```python
from build123d import *

# Parameters (mm, degrees)
BOSS_EXTRUDE1_DEPTH              = 3.7
CUT_EXTRUDE1_DEPTH               = 1.2
CUT_EXTRUDE2_DEPTH               = 2
CUT_EXTRUDE3_DEPTH               = 20.027535968
BOSS_EXTRUDE3_DEPTH              = 5
M2_CLEARANCE_HOLE1_D             = 2.6
CUT_EXTRUDE4_DEPTH               = 1
CHAMFER2_SIZE                    = 0.75
BOSS_EXTRUDE4_DEPTH              = 3
BOSS_EXTRUDE5_START              = 3
BOSS_EXTRUDE5_DEPTH              = 3
CBORE_FOR_M2_5_SHCS1_D           = 3.1
CBORE_FOR_M2_5_SHCS1_CBORE_D     = 5.5
CBORE_FOR_M2_5_SHCS1_CBORE_DEPTH = 1.5
CUT_EXTRUDE6_DEPTH               = 2.5
SKETCH18_R                       = 3.62
CUT_EXTRUDE7_DEPTH               = 1
CBORE_FOR_M2_SHCS1_D             = 2.6
CBORE_FOR_M2_SHCS1_CBORE_D       = 4.4
CBORE_FOR_M2_SHCS1_CBORE_DEPTH   = 1.5
CHAMFER3_SIZE                    = 0.5
BOSS_EXTRUDE8_DEPTH              = 7.5
BOSS_EXTRUDE9_DEPTH              = 6
FILLET1_R                        = 1


with BuildPart() as part:
    # Sketch1 → Boss-Extrude1 (new body)
    with BuildSketch(Plane(origin=(0, -6, 0), x_dir=(-1, 0, 0), z_dir=(0, -1, 0))):
        with BuildLine():
            Line((7.595, 10.65), (-7.595, 10.65))
            ThreePointArc((-7.595, 10.65), (-11.604295449, 8.989295449), (-13.265, 4.98))
            Line((-13.265, 4.98), (-13.265, -7.46))
            ThreePointArc((-13.265, -7.46), (-11.604295449, -11.469295449), (-7.595, -13.13))
            Line((-7.595, -13.13), (7.595, -13.13))
            ThreePointArc((7.595, -13.13), (11.604295449, -11.469295449), (13.265, -7.46))
            Line((13.265, -7.46), (13.265, 4.98))
            ThreePointArc((13.265, 4.98), (11.604295449, 8.989295449), (7.595, 10.65))
        make_face()
    extrude(amount=-BOSS_EXTRUDE1_DEPTH)

    # Sketch3 → Cut-Extrude1 (cut)
    with BuildSketch(Plane(origin=(0, -2.3, 0), x_dir=(1, 0, 0), z_dir=(0, 1, 0))):
        with BuildLine():
            Line((-7.595, -10.48), (7.595, -10.48))
            ThreePointArc((7.595, -10.48), (9.730462479, -9.595462479), (10.615, -7.46))
            Line((10.615, -7.46), (10.615, 4.98))
            ThreePointArc((10.615, 4.98), (9.730462479, 7.115462479), (7.595, 8))
            Line((7.595, 8), (-7.595, 8))
            ThreePointArc((-7.595, 8), (-9.730462479, 7.115462479), (-10.615, 4.98))
            Line((-10.615, 4.98), (-10.615, -7.46))
            ThreePointArc((-10.615, -7.46), (-9.730462479, -9.595462479), (-7.595, -10.48))
        make_face()
    extrude(amount=-CUT_EXTRUDE1_DEPTH, mode=Mode.SUBTRACT)

    # Sketch4 → Cut-Extrude2 (cut)
    with BuildSketch(Plane(origin=(0, -6, 0), x_dir=(1, 0, 0), z_dir=(0, 1, 0))):
        with BuildLine():
            Line((9.25, -4.27), (-9.25, -4.27))
            ThreePointArc((-9.25, -4.27), (-9.603553391, -4.416446609), (-9.75, -4.77))
            Line((-9.75, -4.77), (-9.75, -11.98))
            Line((-9.75, -11.98), (-9.75, -13.13))
            Line((-9.75, -13.13), (9.75, -13.13))
            Line((9.75, -13.13), (9.75, -11.98))
            Line((9.75, -11.98), (9.75, -4.77))
            ThreePointArc((9.75, -4.77), (9.603553391, -4.416446609), (9.25, -4.27))
        make_face()
    extrude(amount=CUT_EXTRUDE2_DEPTH, mode=Mode.SUBTRACT)

    # Sketch5 → Cut-Extrude3 (cut, through all)
    with BuildSketch(Plane(origin=(0, -2.3, 0), x_dir=(1, 0, 0), z_dir=(0, 1, 0))):
        with BuildLine():
            Line((-9.25, -9.63), (9.25, -9.63))
            ThreePointArc((9.25, -9.63), (9.603553391, -9.483553391), (9.75, -9.13))
            Line((9.75, -9.13), (9.75, -4.77))
            ThreePointArc((9.75, -4.77), (9.603553391, -4.416446609), (9.25, -4.27))
            Line((9.25, -4.27), (-9.25, -4.27))
            ThreePointArc((-9.25, -4.27), (-9.603553391, -4.416446609), (-9.75, -4.77))
            Line((-9.75, -4.77), (-9.75, -9.13))
            ThreePointArc((-9.75, -9.13), (-9.603553391, -9.483553391), (-9.25, -9.63))
        make_face()
    extrude(amount=-CUT_EXTRUDE3_DEPTH, mode=Mode.SUBTRACT)

    # Sketch6 → Boss-Extrude3 (add, symmetric)
    with BuildSketch(Plane(origin=(0, 0, 1.24), x_dir=(-1, 0, 0), z_dir=(0, 0, -1))):
        Polygon((-11.94, -2.3), (-11.94, 0.7), (-11.44, 0.7), (-11.44, 1.7), (-12.19, 2.45), (-13.265, 2.45), (-13.265, -2.3), align=None)
    boss_extrude3 = extrude(amount=BOSS_EXTRUDE3_DEPTH, both=True)

    # Mirror1: Boss-Extrude3 across plane
    add(boss_extrude3.mirror(Plane(origin=(0, 0, 0), x_dir=(0, 0, 1), z_dir=(1, 0, 0))))

    # M2 Clearance Hole1 (through all)
    with Locations(Plane(origin=(0, -3.5, 0), x_dir=(1, 0, 0), z_dir=(0, 1, 0))):
        with Locations((-7.615, 5.15), (7.615, 5.15)):
            Hole(M2_CLEARANCE_HOLE1_D / 2)

    # Sketch9 → Cut-Extrude4 (cut)
    with BuildSketch(Plane.XZ.offset(6)):
        Polygon((-7.615, -2.667393842), (-9.765, -3.908696921), (-9.765, -6.391303079), (-7.615, -7.632606158), (-5.465, -6.391303079), (-5.465, -3.908696921), align=None)
        Polygon((7.615, -2.667393842), (5.465, -3.908696921), (5.465, -6.391303079), (7.615, -7.632606158), (9.765, -6.391303079), (9.765, -3.908696921), align=None)
    extrude(amount=-CUT_EXTRUDE4_DEPTH, mode=Mode.SUBTRACT)

    # Chamfer2
    chamfer2_edges = [part.edges().sort_by_distance(p)[0] for p in [
        (-13.265, 2.45, 1.24),
        (13.265, 2.45, 1.24),
    ]]
    chamfer(chamfer2_edges, length=CHAMFER2_SIZE)

    # Sketch11 → Boss-Extrude4 (add)
    with BuildSketch(Plane(origin=(0, 0, -1.76), x_dir=(-1, 0, 0), z_dir=(0, 0, -1))):
        with BuildLine():
            Line((-16.362587065, -18.187498165), (-0.407985075, -19.601950475))
            ThreePointArc((-0.407985075, -19.601950475), (2.579168763, -18.833052112), (4.416654929, -16.355566021))
            Line((4.416654929, -16.355566021), (7.595, -6))
            Line((7.595, -6), (7.595, -3.5))
            Line((7.595, -3.5), (-7.595, -3.5))
            Line((-7.595, -3.5), (-7.595, -11.035213013))
            Line((-7.595, -11.035213013), (-16.362587065, -11.812501835))
            ThreePointArc((-16.362587065, -11.812501835), (-19.28, -15), (-16.362587065, -18.187498165))
        make_face()
    extrude(amount=-BOSS_EXTRUDE4_DEPTH)

    # Sketch12 → Boss-Extrude5 (add)
    with BuildSketch(Plane(origin=(0, 0, -1.76), x_dir=(-1, 0, 0), z_dir=(0, 0, -1)).offset(BOSS_EXTRUDE5_START)):
        with BuildLine():
            Line((-0.407985075, -10.398049525), (-16.362587065, -11.812501835))
            ThreePointArc((-16.362587065, -11.812501835), (-19.28, -15), (-16.362587065, -18.187498165))
            Line((-16.362587065, -18.187498165), (-0.407985075, -19.601950475))
            ThreePointArc((-0.407985075, -19.601950475), (4.62, -15), (-0.407985075, -10.398049525))
        make_face()
    extrude(amount=-BOSS_EXTRUDE5_DEPTH)

    # CBORE for M2.5 SHCS1 (through all)
    with Locations(Plane.XY.offset(1.24)):
        with Locations((0, -15)):
            CounterBoreHole(CBORE_FOR_M2_5_SHCS1_D / 2, CBORE_FOR_M2_5_SHCS1_CBORE_D / 2, CBORE_FOR_M2_5_SHCS1_CBORE_DEPTH)

    # Sketch17 → Cut-Extrude6 (cut)
    with BuildSketch(Plane(origin=(0, 0, -4.76), x_dir=(-1, 0, 0), z_dir=(0, 0, -1))):
        with BuildLine():
            Line((-0.319676617, -11.394142701), (-16.274278607, -12.808595012))
            ThreePointArc((-16.274278607, -12.808595012), (-18.28, -15), (-16.274278607, -17.191404988))
            Line((-16.274278607, -17.191404988), (-0.319676617, -18.605857299))
            ThreePointArc((-0.319676617, -18.605857299), (3.62, -15), (-0.319676617, -11.394142701))
        make_face()
    extrude(amount=-CUT_EXTRUDE6_DEPTH, mode=Mode.SUBTRACT)

    # Sketch18 → Cut-Extrude7 (cut)
    with BuildSketch(Plane(origin=(0, 0, -2.26), x_dir=(-1, 0, 0), z_dir=(0, 0, -1))):
        with Locations((0, -15)):
            Circle(SKETCH18_R)
    extrude(amount=-CUT_EXTRUDE7_DEPTH, mode=Mode.SUBTRACT)

    # CBORE for M2 SHCS1 (through all)
    with Locations(Plane.XY.offset(1.24)):
        with Locations((14.625, -15)):
            CounterBoreHole(CBORE_FOR_M2_SHCS1_D / 2, CBORE_FOR_M2_SHCS1_CBORE_D / 2, CBORE_FOR_M2_SHCS1_CBORE_DEPTH)

    # Chamfer3
    chamfer3_edges = [part.edges().sort_by_distance(p)[0] for p in [
        (6.54, -6, -3.288045382),
        (8.69, -6, -3.288045382),
        (5.465, -6, -5.15),
        (9.765, -6, -5.15),
        (6.54, -6, -7.011954618),
        (8.69, -6, -7.011954618),
        (-8.69, -6, -3.288045382),
        (-6.54, -6, -3.288045382),
        (-9.765, -6, -5.15),
        (-5.465, -6, -5.15),
        (-8.69, -6, -7.011954618),
        (-6.54, -6, -7.011954618),
    ]]
    chamfer(chamfer3_edges, length=CHAMFER3_SIZE)

    # Sketch30 → Boss-Extrude8 (add, symmetric)
    with BuildSketch(Plane(origin=(0, 0, 0), x_dir=(0, 0, -1), z_dir=(1, 0, 0))):
        Polygon((-5.55, -7.7), (-6.4, -9.05), (-6.4, -10.15), (-5.55, -11), (-3.77, -11), (-3.77, -3.5), (-5.55, -3.5), align=None)
    extrude(amount=BOSS_EXTRUDE8_DEPTH, both=True)

    # Sketch31 → Boss-Extrude9 (add)
    with BuildSketch(Plane.XY.offset(1.24)):
        Polygon((8.393841653, -11.106034173), (10.386028006, -11.282651089), (10.562644921, -9.290464736), (14.547017627, -9.643698567), (14.370400712, -11.63588492), (16.362587065, -11.812501835), (16.715820896, -7.828129129), (8.747075483, -7.121661467), align=None)
    extrude(amount=-BOSS_EXTRUDE9_DEPTH)

    # Fillet1
    fillet1_edges = [part.edges().sort_by_distance(p)[0] for p in [
        (8.747075483, -7.121661467, -1.76),
        (16.715820896, -7.828129129, -1.76),
    ]]
    fillet(fillet1_edges, radius=FILLET1_R)


solid = part.part
```
Geometry check sheet. Reference: the model listing, model coordinates, mm. A direction names the side the tool comes from. Coordinates: 2 decimals unless noted, no trailing zeros. Loops run counter-clockwise (first coordinate to the right, second up) from the corner with the lowest first, then second, coordinate; pieces in that order, holes last. Notation, with made-up numbers: (-16.75, 17) -> (7.25, 17) arc R11 ccw to (7.25, 35) -> close; hole circle Ø10 at (54.5, -8). An arc over 180 degrees is marked (long way). Put each result on its own line as item: value.
1) Cross-section at A-A on y = -15.75. Record the boundary of the cut face in (x, z).
Result set:
outline: (-4.6, -1.76) -> (-4.56, -1.76) -> (-4.56, -4.76) -> (-3.54, -4.76) -> (-3.54, -1.26) -> (-1.36, -1.26) -> (-1.36, -0.26) -> (-2.65, -0.26) -> (-2.65, 1.24) -> (-4.6, 1.24) -> close; (1.36, -1.26) -> (3.54, -1.26) -> (3.54, -2.26) -> (13.56, -2.26) -> (13.56, -0.26) -> (12.56, -0.26) -> (12.56, 1.24) -> (2.65, 1.24) -> (2.65, -0.26) -> (1.36, -0.26) -> close; (15.69, -2.26) -> (18.15, -2.26) -> (18.15, -4.76) -> (19.19, -4.76) -> (19.19, 1.24) -> (16.69, 1.24) -> (16.69, -0.26) -> (15.69, -0.26) -> close
2) Thickness scan on line 1 (Y direction, x = 0, z = -3.3); line 2 (X direction, y = -4.05, z = -5.15) (3 decimals); line 3 (Z direction, x = 6.5, y = -9.75). Record the ranges inside material, lowest first.
Result set:
line 1: y = -19.62 to -18.62, -11.38 to -10.38, -6 to -3.5
line 2: x = -13.262 to -8.915, -6.315 to 6.315, 8.915 to 13.262
line 3: z = -1.76 to 1.24, 3.77 to 6.4
3) Release check for a two-part mould opening along X. For faces 6 (the flat face through (2, -15, -0.26)), 7 (the flat face through (9, -12, -4.76)), 8 (the cylindrical face through (16.391, -8.086, -1.802)), 9 (the flat face through (-5.984, -11.25, -0.281)) record: released by +X, released by -X, zero draft, split by the parting line, or undercut.
Result set:
face 6: undercut
face 7: zero draft
face 8: released by +X
face 9: released by -X
4) Tool access check on faces 1 (the cylindrical face through (9, -7.45, -1.8)), 2 (the flat face through (6.555, -5.254, -3.279)), 3 (the cylindrical face through (16.66, -15.84, 0.5)), 4 (the flat face through (8, -5, 4.27)), 5 (the flat face through (-6.52, -5.25, -3.3)). Record the directions out of +Z, -Z, +X, -X, +Y, -Y that give a thin tool (end or side, any length) a straight path to the whole face; none if there is none.
Result set:
face 1: +Z, -Z
face 2: none
face 3: +Z
face 4: +Y, -Y
face 5: -Y
5) Gauge pin test, flat ends, axial feed: pin 1 Ø3.5 at (x, y) = (15, -16) entering from +Z; pin 2 Ø8 at (x, z) = (-6, -5) entering from +Y; pin 3 Ø3.5 at (x, y) = (7.5, -14) entering from -Z; pin 4 Ø1.5 at (y, z) = (-16, 2.5) entering from -X. Record the tip position at first contact, or that the pin passes through.
Result set:
pin 1: stops at z = 1.24
pin 2: stops at y = -2.3
pin 3: stops at z = -2.26
pin 4: passes through
6) Cross-section at B-B on x = 17.5. Record the boundary of the cut face in (y, z).
Result set:
outline: (-17.87, -4.76) -> (-16.68, -4.76) -> (-16.68, -2.26) -> (-13.32, -2.26) -> (-13.32, -4.76) -> (-12.13, -4.76) -> (-12.13, 1.24) -> (-17.87, 1.24) -> close
